Here's how the part is built. I have some questions about the finished solid (model axes, mm). Face numbers are marked on the shaded views. A direction names the side the tool comes from. Give positions to 0.01 mm unless a question says otherwise; leave off trailing zeros. Loops run counter-clockwise (first coordinate to the right, second up) from the corner with the lowest first, then second, coordinate; pieces in that order, holes last. Notation, with made-up numbers: M 32.25,54.5 L 42.25,54.5 A17 ccw 42.25,75.5 Z; hole C 68,-2 d10. An arc over 180 degrees is marked long. Answer as CSV lines item,"result". Start each with the question number.
Item 1: I want a section at A-A on y = 10. List the corners of the cut face in (x, z) for me, plus the area to 3 significant figures.
Item 2: I want a section at B-B on x = 22. List the corners of the cut face in (y, z) for me, plus the area to 3 significant figures.
Item 3: I want a section at D-D on z = -33. List the corners of the cut face in (x, y) for me, plus the area to 3 significant figures.
Item 4: I want a section at C-C on z = -6. List the corners of the cut face in (x, y) for me.
Item 5: If I drill on line 1 along X through (y, z) = (1.55, -6); line 2 along Z through (x, y) = (21.5, 2); line 3 along Y through (x, z) = (32, -60), over which ranges is the centre line in solid material (lowest first)? Write a range as from..to.
Item 6: For the marked faces 1 and 2, which set-ups out of +Z, -Z, +X, -X, +Y, -Y let a thin tool reach every point of the face, with its end or its side?
Item 7: Will these pins go through, and if not, where does the flat tip stop? P1, Ø13.5, axis at x = 19, z = -45, coming from the +Y side; P2, Ø5.5, axis at y = 10, z = -33, coming from the -X side.
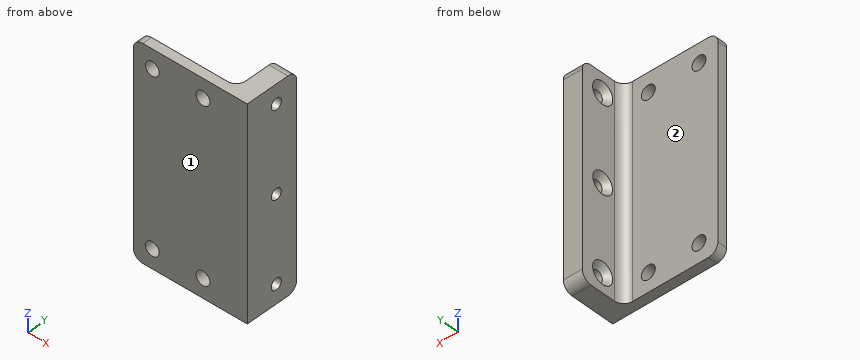
from build123d import *

# Parameters (mm, degrees)
SKETCH1_W           = 36
SKETCH1_H           = 66
SKETCH1_R           = 2.2
BOSS_EXTRUDE1_DEPTH = 3
SKETCH2_W           = 6
SKETCH2_H           = 66
BOSS_EXTRUDE2_DEPTH = 14
SKETCH3_R           = 1.7
SKETCH3_R_2         = 1.752037124
CUT_EXTRUDE1_DEPTH  = 75.464756765
CHAMFER1_SIZE       = 1.7
FILLET1_R           = 3


with BuildPart() as part:
    # Sketch1 → Boss-Extrude1 (new body)
    with BuildSketch(Plane(origin=(0, 0, 0), x_dir=(1, 0, 0), z_dir=(0, 1, 0))):
        with Locations((18, 33)):
            Rectangle(SKETCH1_W, SKETCH1_H)
        with Locations(Location((6, 60, 0), (0, 0, 270))):
            Circle(SKETCH1_R, mode=Mode.SUBTRACT)
        with Locations(Location((6, 6, 0), (0, 0, 90))):
            Circle(SKETCH1_R, mode=Mode.SUBTRACT)
        with Locations(Location((22, 6, 0), (0, 0, 270))):
            Circle(SKETCH1_R, mode=Mode.SUBTRACT)
        with Locations(Location((22, 60, 0), (0, 0, 90))):
            Circle(SKETCH1_R, mode=Mode.SUBTRACT)
    extrude(amount=BOSS_EXTRUDE1_DEPTH)

    # Sketch2 → Boss-Extrude2 (add)
    with BuildSketch(Plane(origin=(0, 3, 0), x_dir=(1, 0, 0), z_dir=(0, 1, 0))):
        with Locations((33, 33)):
            Rectangle(SKETCH2_W, SKETCH2_H)
    extrude(amount=BOSS_EXTRUDE2_DEPTH)

    # Sketch3 → Cut-Extrude1 (cut, through all)
    with BuildSketch(Plane.ZY.offset(-30)):
        with Locations((-33, 10)):
            Circle(SKETCH3_R)
        with Locations((-6, 10)):
            Circle(SKETCH3_R_2)
        with Locations(Location((-60, 10, 0), (0, 0, 180))):
            Circle(SKETCH3_R_2)
    extrude(amount=-CUT_EXTRUDE1_DEPTH, mode=Mode.SUBTRACT)

    # Chamfer1
    chamfer1_edges = [part.edges().sort_by_distance(p)[0] for p in [
        (30, 10, -58.247962876),
        (30, 10, -7.752037124),
        (30, 10, -34.7),
    ]]
    chamfer(chamfer1_edges, length=CHAMFER1_SIZE)

    # Fillet1
    fillet1_edges = [part.edges().sort_by_distance(p)[0] for p in [
        (30, 3, -33),
        (33, 17, -66),
        (33, 17, 0),
        (0, 1.5, -66),
        (0, 1.5, 0),
    ]]
    fillet(fillet1_edges, radius=FILLET1_R)


solid = part.part
Result:
1,outline,"M 30,-66 L 36,-66 L 36,-61.75 L 31.7,-61.75 L 30,-63.45 Z; M 30,-56.55 L 31.7,-58.25 L 36,-58.25 L 36,-34.7 L 31.7,-34.7 L 30,-36.4 Z; M 30,-29.6 L 31.7,-31.3 L 36,-31.3 L 36,-7.75 L 31.7,-7.75 L 30,-9.45 Z; M 30,-2.55 L 31.7,-4.25 L 36,-4.25 L 36,0 L 30,0 Z"
1,area,"325 mm^2"
2,outline,"M 0,-66 L 3,-66 L 3,-62.2 L 0,-62.2 Z; M 0,-57.8 L 3,-57.8 L 3,-8.2 L 0,-8.2 Z; M 0,-3.8 L 3,-3.8 L 3,0 L 0,0 Z"
2,area,"172 mm^2"
3,outline,"M 0,0 L 36,0 L 36,8.3 L 31.7,8.3 L 30,6.6 L 30,6 A3 cw 27,3 L 0,3 Z; M 30,13.4 L 31.7,11.7 L 36,11.7 L 36,17 L 30,17 Z"
3,area,"171 mm^2"
4,outline,"M 0,0 L 3.8,0 L 3.8,3 L 0,3 Z; M 8.2,0 L 19.8,0 L 19.8,3 L 8.2,3 Z; M 24.2,0 L 36,0 L 36,8.25 L 31.7,8.25 L 30,6.55 L 30,6 A3 cw 27,3 L 24.2,3 Z; M 30,13.45 L 31.7,11.75 L 36,11.75 L 36,17 L 30,17 Z"
5,line 1,"0..3.8, 8.2..19.8, 24.2..36"
5,line 2,"-66..-62.14, -57.86..-8.14, -3.86..0"
5,line 3,"0..8.25, 11.75..17"
6,face 1,"+Z, -Z, +X, -X, -Y"
6,face 2,"+Z, -Z, -X, +Y"
7,P1,"y = 3"
7,P2,"x = 30.65"
